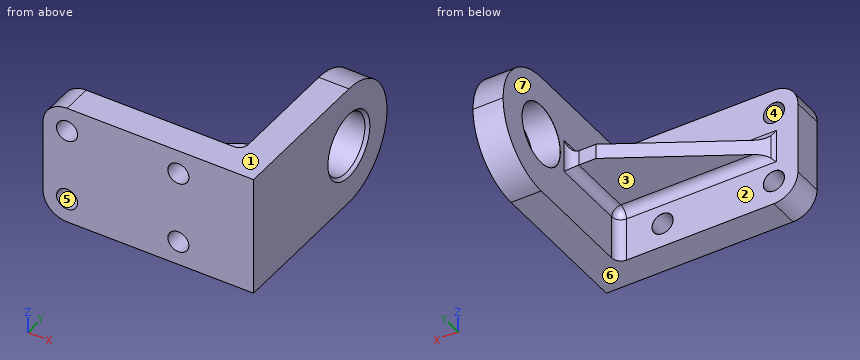
from build123d import *

# Parameters (mm, degrees)
RESSALTO_EXTRUS_O1_DEPTH             = 20
FILETE1_R                            = 8
FILETE2_R                            = 20
FILETE3_R                            = 3
NERVURA23_START                      = -2.5
NERVURA23_DEPTH                      = 5
FILETE4_R                            = 3
FURO_DE_DI_METRO_7_0_7_1_D           = 7
FURO_DE_DI_METRO_7_0_7_1_CSINK_D     = 7.05
FURO_DE_DI_METRO_7_0_7_1_CSINK_ANGLE = 90


# Read off the part's stored shape, not the designer's step: Nervura23
with BuildPart() as part:
    # Esboço1 → Ressalto-extrusão1 (new, symmetric)
    with BuildSketch(Plane.XY):
        Polygon((0, 0), (70, 0), (70, 70), (60, 70), (60, 10), (0, 10), align=None)
    extrude(amount=RESSALTO_EXTRUS_O1_DEPTH, both=True)

    # Filete1
    filete1_edges = [part.edges().sort_by_distance(p)[0] for p in [
        (0, 5, -20),
        (0, 5, 20),
    ]]
    fillet(filete1_edges, radius=FILETE1_R)

    # Filete2
    filete2_edges = [part.edges().sort_by_distance(p)[0] for p in [
        (65, 70, 20),
        (65, 70, -20),
    ]]
    fillet(filete2_edges, radius=FILETE2_R - 0.0001)  # a hair under: the kernel refuses the full size

    # Filete3
    filete3_edges = [part.edges().sort_by_distance(p)[0] for p in [
        (60, 10, 0),
    ]]
    fillet(filete3_edges, radius=FILETE3_R)

    # Nervura23 outline → Nervura23 (add)
    with BuildSketch(Plane.XY.offset(NERVURA23_START)):
        with BuildLine():
            Line((60, 35), (51.301270189, 35))
            Line((51.301270189, 35), (8, 10))
            Line((8, 10), (57, 10))
            ThreePointArc((57, 10), (59.121320344, 10.878679656), (60, 13))
            Line((60, 13), (60, 35))
        make_face()
    extrude(amount=NERVURA23_DEPTH)

    # Filete4
    filete4_edges = [part.edges().sort_by_distance(p)[0] for p in [
        (59.121320344, 10.878679656, -2.5),
        (59.121320344, 10.878679656, 2.5),
        (8, 10, 0),
        (60, 35, 0),
        (32.5, 10, -2.5),
        (60, 24, -2.5),
        (32.5, 10, 2.5),
        (60, 24, 2.5),
    ]]
    fillet(filete4_edges, radius=FILETE4_R)

    # Furo de diâmetro Ø7.0 (7)1 (through all)
    with Locations(Plane(origin=(0, 10, 0), x_dir=(1, 0, 0), z_dir=(0, 1, 0))):
        with Locations((8, 12), (8, -12), (45, 12), (45, -12)):
            CounterSinkHole(FURO_DE_DI_METRO_7_0_7_1_D / 2, FURO_DE_DI_METRO_7_0_7_1_CSINK_D / 2, counter_sink_angle=FURO_DE_DI_METRO_7_0_7_1_CSINK_ANGLE)

    # Esboço11 → Furo de diâmetro Ø20.0 (20)1 (revolve, cut)
    with BuildSketch(Plane(origin=(70, 50, 0), x_dir=(0, 0, -1), z_dir=(0, 1, 0))):
        Polygon((0, 0), (0, 10), (10.025, 10), (10, 9.975), (10, 1), (11, 0), align=None)
    revolve(axis=Axis((76.35, 50, 0), (-1, 0, 0)), mode=Mode.SUBTRACT)


solid = part.part
Read the model definition and answer for the solid it produces. Units are mm, in the model's axes. Face numbers are marked on the shaded views. A direction names the side the tool comes from. Round coordinates to 2 decimals unless told otherwise and drop trailing zeros. Write each loop counter-clockwise with the first axis right and the second up, starting at its lowest first coordinate (ties: lowest second). Pieces come first, ordered by that corner, then holes. Notation, with made-up numbers: (40.25, 54.5) - (99.25, 54.5) arc R12 ccw to (99.25, 74.5) - close; hole circle Ø11 at (15, 67). An arc over 180 degrees is marked (long way). Use a Markdown table: item, result.
(1) The part is cut by section A-A (y = 5.5). Write down the section's boundary in (x, z), then the cut area to 3 significant figures.
Reported:
| item | result |
|---|---|
| outline | (0, -12) arc R8 ccw to (8, -20) - (70, -20) - (70, 20) - (8, 20) arc R8 ccw to (0, 12) - close; hole circle Ø7 at (8, -12); hole circle Ø7 at (8, 12); hole circle Ø7 at (45, -12); hole circle Ø7 at (45, 12) |
| area | 2,620 mm2 |
(2) Each of these flat-tipped pins is pushed along its axis until it touches: pin 1 Ø2.5 at (x, z) = (53, 0.5) entering from +Y; pin 2 Ø6 at (x, z) = (25, -10) entering from +Y; pin 3 Ø11 at (x, y) = (29, 24.5) entering from +Z; pin 4 Ø5.5 at (x, z) = (45, -12) entering from -Y. Where does it stop, or does it pass through?
Reported:
| item | result |
|---|---|
| pin 1 | y = 35 |
| pin 2 | y = 10 |
| pin 3 | z = 2.5 |
| pin 4 | through |
(3) Which of the six approach directions +Z, -Z, +X, -X, +Y, -Y give full straight-line access (tool end or side, diameter ignored) to the marked faces 1, 2 and 3?
Reported:
| item | result |
|---|---|
| face 1 | +Z, +X, -X, +Y, -Y |
| face 2 | -X, +Y |
| face 3 | -Z, -X, +Y |
(4) The part is cut by section B-B (x = 45). Write down the section's boundary in (y, z) (3 decimals), then the cut area to 3 significant figures.
Reported:
| item | result |
|---|---|
| outline | (0, -20) - (10, -20) - (10, -15.525) - (9.975, -15.5) - (0, -15.5) - close; (0, -8.5) - (9.975, -8.5) - (10, -8.475) - (10, -5.5) arc R3 cw to (13, -2.5) - (31.362, -2.5) - (31.362, 2.5) - (13, 2.5) arc R3 cw to (10, 5.5) - (10, 8.475) - (9.975, 8.5) - (0, 8.5) - close; (0, 15.5) - (9.975, 15.5) - (10, 15.525) - (10, 20) - (0, 20) - close |
| area | 371 mm2 |
(5) The part is cut by section D-D (y = 27). Write down the section's boundary in (x, z), then the cut area to 3 significant figures.
Reported:
| item | result |
|---|---|
| outline | (37.44, -2.5) - (57, -2.5) arc R3 cw to (60, -5.5) - (60, -20) - (70, -20) - (70, 20) - (60, 20) - (60, 5.5) arc R3 cw to (57, 2.5) - (37.44, 2.5) - close |
| area | 517 mm2 |
(6) The part is cut by section C-C (x = 26.5). Write down the section's boundary in (y, z).
Reported:
| item | result |
|---|---|
| outline | (0, -20) - (10, -20) - (10, -5.5) arc R3 cw to (13, -2.5) - (20.68, -2.5) - (20.68, 2.5) - (13, 2.5) arc R3 cw to (10, 5.5) - (10, 20) - (0, 20) - close |
(7) Straight lines are drawn through the part: line 1 along X through (y, z) = (6.75, -12); line 2 along Z through (x, y) = (63.75, 50); line 3 along Z through (x, y) = (45, 3). For each, find the intervals that lie inside material, in ascending order. Write a range as [from, to].
Reported:
| item | result |
|---|---|
| line 1 | [0, 4.5], [11.5, 41.5], [48.5, 70] |
| line 2 | [-20, -10], [10, 20] |
| line 3 | [-20, -15.5], [-8.5, 8.5], [15.5, 20] |
(8) The mould has two halves that part along X. Classify the marked faces 4, 5, 6 and 7: released by +X, released by -X, zero draft, split by the parting line, or undercut.
Reported:
| item | result |
|---|---|
| face 4 | undercut |
| face 5 | undercut |
| face 6 | zero draft |
| face 7 | released by -X |
